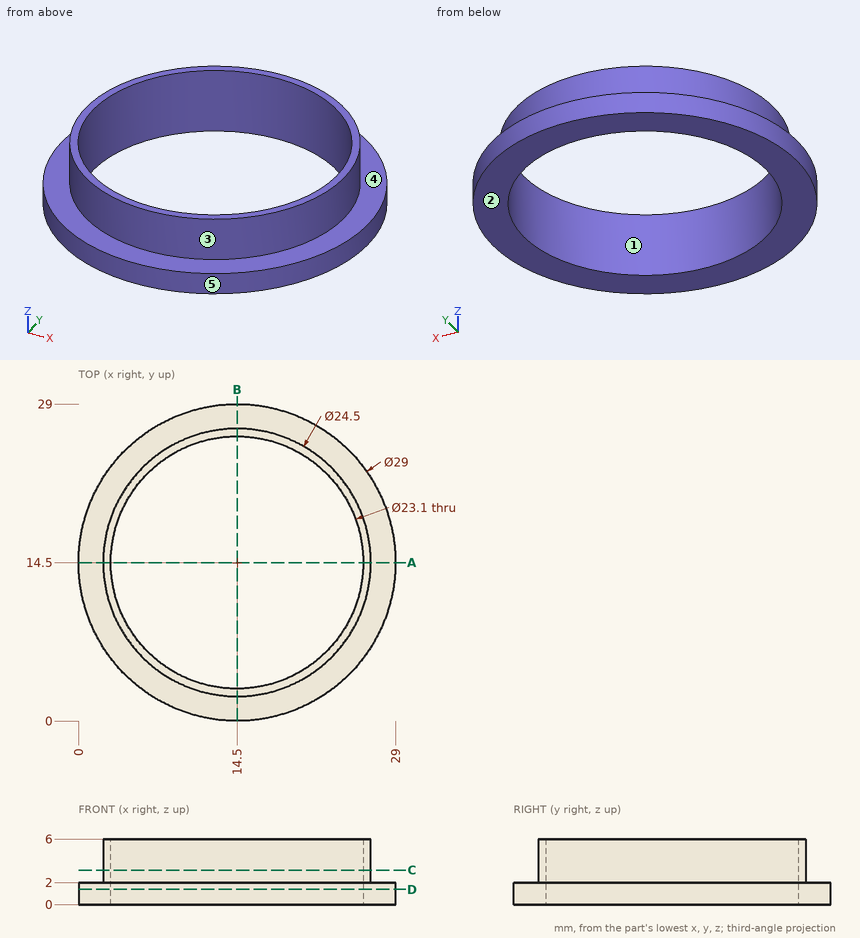
Design review of the part shown in the three views and the two pictorial views. Dimensions are in mm from the part's minimum x, y and z. A direction names the side the tool comes from. Give positions to 0.01 mm unless a question says otherwise; leave off trailing zeros. Loops run counter-clockwise (first coordinate to the right, second up) from the corner with the lowest first, then second, coordinate; pieces in that order, holes last. Notation, with made-up numbers: M 72,-1 L 106,-1 A32 cw 106,35 Z; hole C 71,35 d4. An arc over 180 degrees is marked long. Answer as a JSON object with one key per item and string values.
Item 1: We need section A-A (y = 14.5). State the section outline as (x, z) points, and give its area (3 significant figures).
Output values:
{"outline": "M 0,0 L 2.95,0 L 2.95,6 L 2.25,6 L 2.25,2 L 0,2 Z; M 26.05,0 L 29,0 L 29,2 L 26.75,2 L 26.75,6 L 26.05,6 Z", "area": "17.4 mm2"}
Item 2: For P1, Ø3, axis at x = 20.5, z = 2.5, coming from the +Y side, flat-tipped, find the tip position at first contact; note if it passes through.
Output values:
{"P1": "stops at y = 28.26"}
Item 3: Mouldability with a two-part tool opening along Y and no side actions: class the marked faces 1, 2 and 3 as pulls with the +Y half, pulls with the -Y half, needs draft (parallel to the pull), parting line crosses it, or undercut.
Output values:
{"face 1": "undercut", "face 2": "needs draft", "face 3": "parting line crosses it"}
Item 4: We need section D-D (z = 1.4). State the section outline as (x, y) points.
Output values:
{"outline": "C 14.5,14.5 d29; hole C 14.5,14.5 d23.1"}
Item 5: We need section C-C (z = 3.15). State the section outline as (x, y) points.
Output values:
{"outline": "C 14.5,14.5 d24.5; hole C 14.5,14.5 d23.1"}
Item 6: Machinability: for the marked faces 4 and 5, which of the approach directions +Z, -Z, +X, -X, +Y, -Y give a long, thin tool a straight path to every point of the face, cutting with its end or side? Answer none if there is none.
Output values:
{"face 4": "+Z", "face 5": "+Z, -Z"}
Item 7: Wall thickness on line 1 along Y through (x, z) = (14.5, 2.9); line 2 along Y through (x, z) = (14.25, 1.8); line 3 along X through (y, z) = (19, 4.7): over which ranges is each line inside the solid? List them lowest first.
Output values:
{"line 1": "y = 2.25 to 2.95, 26.05 to 26.75", "line 2": "y = 0 to 2.95, 26.05 to 29", "line 3": "x = 3.11 to 3.86, 25.14 to 25.89"}
